Geometry check sheet. Reference: the model listing, model coordinates, mm. A direction names the side the tool comes from. Give positions to 0.01 mm unless a question says otherwise; leave off trailing zeros. Order: outer loops, then holes, each group sorted by start corner. A loop starts at its lowest first (then second) coordinate and runs counter-clockwise, first axis right, second up. Notation, with made-up numbers: M 78.5,-1.5 L 136.5,-1.5 A18 ccw 136.5,31.5 Z; hole C -1.5,49 d3. An arc over 180 degrees is marked long. Answer as CSV lines item,"result". Start each with the question number.
Q1. Section check D-D, the plane y = 626. Record the boundary of the cut face in (x, z), then the cut area to 3 significant figures.
Q2. Section check A-A, the plane x = 0. Record the boundary of the cut face in (y, z).
Q3. Go/stop test with flat-tipped pins: pin 1 (1.5 mm diameter, centred on x = -149.5, y = 789, fed in from -Z); pin 2 (4 mm diameter, centred on x = 296, z = 155.5, fed in from -Y); pin 3 (1.5 mm diameter, centred on x = -168.5, z = 568.5, fed in from +Y). Record where each tip stops, or that it passes through.
Q4. Section check B-B, the plane y = -157. Record the boundary of the cut face in (x, z), then the cut area to 3 significant figures.
Q5. Thickness scan on line 1 (Z direction, x = -378, y = -76.5); line 2 (Y direction, x = 0, z = -569); line 3 (X direction, y = 868, z = -25). Record the ranges inside material, lowest first.
Q6. Mould release check, pull along Z, two halves, no side actions. Record for faces 4 (the cylindrical face through (61.036, 796.011, 168.417)), 5 (the flat face through (106, 233, -889)), 6 (the cylindrical face through (-11.171, -507.877, -688.645)): +Z half, -Z half, draft (parallel to the pull), parting line (faces both ways), or undercut.
Q7. Set-up check for faces 1 (the flat face through (-383, 0, -7)), 2 (the flat face through (-3, 508, -28)), 3 (the cylindrical face through (-11.171, -507.877, 688.645)): record each of +Z, -Z, +X, -X, +Y, -Y from which the full face is reachable in a straight line by a thin tool's end or side.
Q8. Section check C-C, the plane z = -704.5. Record the boundary of the cut face in (x, y), then the cut area to 3 significant figures.
```python
from build123d import *

# Parameters (mm, degrees)
SKETCH1_W           = 1016
SKETCH1_H           = 1778
BOSS_EXTRUDE1_DEPTH = 508
SKETCH2_R           = 508
SKETCH2_R_2         = 203.2
BOSS_EXTRUDE2_DEPTH = 584.2
SKETCH3_R           = 508
BOSS_EXTRUDE3_DEPTH = 406.4
CUT_EXTRUDE1_REACH  = 2149.615
SKETCH5_R           = 254


with BuildPart() as part:
    # Sketch1 → Boss-Extrude1 (new body)
    with BuildSketch(Plane(origin=(0, 0, 0), x_dir=(1, 0, 0), z_dir=(0, 1, 0))):
        Rectangle(SKETCH1_W, SKETCH1_H)
    extrude(amount=BOSS_EXTRUDE1_DEPTH)

    # Sketch2 → Boss-Extrude2 (add)
    with BuildSketch(Plane(origin=(0, 508, 0), x_dir=(1, 0, 0), z_dir=(0, 1, 0))):
        with Locations(Location((0, 25.4, 0), (0, 0, 180))):
            Circle(SKETCH2_R)
        with Locations(Location((0, 25.4, 0), (0, 0, 270))):
            Circle(SKETCH2_R_2, mode=Mode.SUBTRACT)
    extrude(amount=BOSS_EXTRUDE2_DEPTH)

    # Sketch3 → Boss-Extrude3 (add)
    with BuildSketch(Plane.XY.offset(889)):
        Circle(SKETCH3_R)
    boss_extrude3 = extrude(amount=-BOSS_EXTRUDE3_DEPTH)

    # Sketch5 → Cut-Extrude1 (cut, up to next)
    with BuildSketch(Plane.XY.offset(889), mode=Mode.PRIVATE) as cut_extrude1_sk1:
        Circle(SKETCH5_R)
    cut_extrude1_tool1 = extrude(cut_extrude1_sk1.sketch, amount=-CUT_EXTRUDE1_REACH, mode=Mode.PRIVATE) & part.part
    cut_extrude1 = cut_extrude1_tool1.solids().sort_by_distance((0, 0, 889))[0]
    add(cut_extrude1, mode=Mode.SUBTRACT)

    # Mirror1: Boss-Extrude3, Cut-Extrude1 across plane
    add(boss_extrude3.mirror(Plane.XY))
    add(cut_extrude1.mirror(Plane.XY), mode=Mode.SUBTRACT)


solid = part.part
```
Answer block:
1,outline,"C 0,-25.4 d1016; hole C 0,-25.4 d406.4"
1,area,"681,000 mm2"
2,outline,"M -508,-889 L -254,-889 L -254,-482.6 L -508,-482.6 Z; M -508,482.6 L -254,482.6 L -254,889 L -508,889 Z; M 254,-889 L 508,-889 L 508,-533.4 L 1092.2,-533.4 L 1092.2,-228.6 L 508,-228.6 L 508,177.8 L 1092.2,177.8 L 1092.2,482.6 L 508,482.6 L 508,889 L 254,889 Z"
3,pin 1,"stops at z = -511.13"
3,pin 2,"stops at y = 0"
3,pin 3,"stops at y = 508"
4,outline,"M -483.13,-889 L -199.67,-889 L -199.67,-482.6 L -483.13,-482.6 Z; M -483.13,482.6 L -199.67,482.6 L -199.67,889 L -483.13,889 Z; M 199.67,-889 L 483.13,-889 L 483.13,-482.6 L 199.67,-482.6 Z; M 199.67,482.6 L 483.13,482.6 L 483.13,889 L 199.67,889 Z"
4,area,"461,000 mm2"
5,line 1,"z = -889 to -482.6, 482.6 to 889"
5,line 2,"y = -508 to -254, 254 to 508"
5,line 3,"x = -508 to -203.2, 203.2 to 508"
6,face 4,"undercut"
6,face 5,"-Z half"
6,face 6,"draft"
7,face 1,"+X, -X, -Y"
7,face 2,"+Y"
7,face 3,"+Z, -Z, -Y"
8,outline,"M -508,0 A508 ccw 508,0 L 508,508 L -508,508 Z; hole C 0,0 d508"
8,area,"719,000 mm2"
